Design review of the part built by this model. Coordinates are the model's own, in mm. Face numbers are marked on the shaded views. A direction names the side the tool comes from. Round coordinates to 2 decimals unless told otherwise and drop trailing zeros. Loops run counter-clockwise (first coordinate to the right, second up) from the corner with the lowest first, then second, coordinate; pieces in that order, holes last. Notation, with made-up numbers: (81.5, 60.25) - (96.5, 60.25) arc R23 cw to (96.5, 97.25) - close; hole circle Ø8 at (-38, 45). An arc over 180 degrees is marked (long way). Answer as CSV lines item,"result". Start each with the question number.
(1) For the marked faces 4 and 5, list the 3-axis set-ups (+Z, -Z, +X, -X, +Y, -Y) from which the entire face can be reached by the end or side of a thin tool; tool diameter is ignored.
(2) Consider section C-C (y = 1). Give the boundary of the cut face in (x, z) (3 decimals).
(3) Consider section D-D (x = 3.25). Give the boundary of the cut face in (y, z).
(4) For P1, Ø4, axis at x = 0, z = 0, coming from the +Y side (1 decimal); P2, Ø3, axis at x = -2, y = 5, coming from the -Z side; P3, Ø8, axis at x = 6, y = 6, coming from the +Z side; P4, Ø2, axis at x = 5, y = 12, coming from the +Z side, all flat-tipped, find the tip position at first contact; note any pin that passes through.
(5) Consider section B-B (z = 0). Give the boundary of the cut face in (x, y) (3 decimals).
(6) Mouldability with a two-part tool opening along Z and no side actions: class the marked faces 1, 2 and 3 as released by +Z, released by -Z, zero draft, split by the parting line, or undercut.
(7) Wall thickness on L1, parallel to Z at x = 0, y = 7 (3 decimals); L2, parallel to Y at x = -6.5, z = -4: over which ranges is each line inside the solid? List them lowest first.
(8) Consider section A-A (x = 0). Give the boundary of the cut face in (y, z) (3 decimals), and give its area (3 significant figures).
Autodesk Inventor part; units mm, degrees
ref_plane "YZ Plane" through (0, 0, 0) normal (1, 0, 0) x (0, 1, 0)
ref_plane "XZ Plane" through (0, 0, 0) normal (0, 1, 0) x (-1, 0, 0)
ref_plane "XY Plane" through (0, 0, 0) normal (0, 0, 1) x (1, 0, 0)
sketch "Sketch1" plane through (0, 0, 0) normal (0, 1, 0) x (-1, 0, 0)
  circle A0 centre (0, 0) radius 9
  dimension "d0" = 18
extrude "Extrusion1" add sketch "Sketch1" along normal blind 1.5
sketch "Sketch2" plane through (0, 1.5, 0) normal (0, 1, 0) x (1, 0, 0)
  circle A0 centre (0, 0) radius 6.05
  dimension "d3" = 12.1
extrude "Extrusion2" add sketch "Sketch2" along normal blind 11.2
sketch "Sketch3" plane through (0, 12.7, 0) normal (0, 1, 0) x (1, 0, 0)
  circle A0 centre (0, 0) radius 9
  dimension "d6" = 18
extrude "Extrusion3" add sketch "Sketch3" along normal blind 1.5
sketch "Sketch4" plane through (0, 14.2, 0) normal (0, 1, 0) x (1, 0, 0)
  circle A0 centre (0, 0) radius 6.05
  circle A1 centre (0, 0) radius 2.625
  dimension "d9" = 5.25
extrude "Extrusion4" cut sketch "Sketch4" against normal through all contours A1
properties part number "10mm_Idle_Pulley"
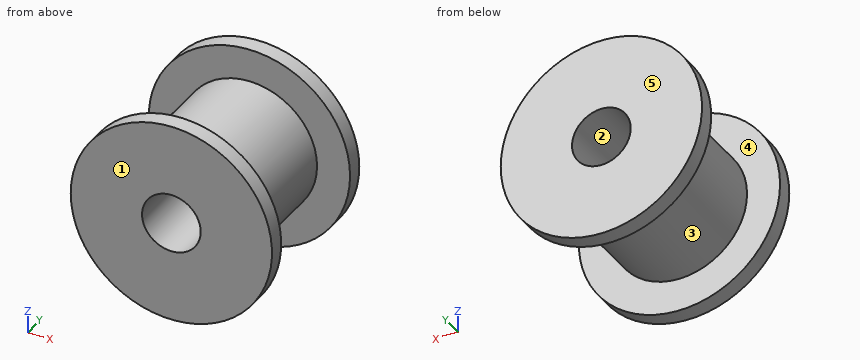
Determined:
1,face 4,"none"
1,face 5,"+Z, -Z, +X, -X, +Y"
2,outline,"circle Ø18 at (0, 0); hole circle Ø5.25 at (0, 0)"
3,outline,"(0, -8.39) - (1.5, -8.39) - (1.5, -5.1) - (12.7, -5.1) - (12.7, -8.39) - (14.2, -8.39) - (14.2, 8.39) - (12.7, 8.39) - (12.7, 5.1) - (1.5, 5.1) - (1.5, 8.39) - (0, 8.39) - close"
4,P1,"passes through"
4,P2,"stops at z = -6.03"
4,P3,"stops at z = 5.71"
4,P4,"stops at z = 7.91"
5,outline,"(-9, 0) - (-2.625, 0) - (-2.625, 14.2) - (-9, 14.2) - (-9, 12.7) - (-6.05, 12.7) - (-6.05, 1.5) - (-9, 1.5) - close; (2.625, 0) - (9, 0) - (9, 1.5) - (6.05, 1.5) - (6.05, 12.7) - (9, 12.7) - (9, 14.2) - (2.625, 14.2) - close"
6,face 1,"zero draft"
6,face 2,"undercut"
6,face 3,"split by the parting line"
7,L1,"z = -6.05 to -2.625, 2.625 to 6.05"
7,L2,"y = 0 to 1.5, 12.7 to 14.2"
8,outline,"(0, -9) - (1.5, -9) - (1.5, -6.05) - (12.7, -6.05) - (12.7, -9) - (14.2, -9) - (14.2, -2.625) - (0, -2.625) - close; (0, 2.625) - (14.2, 2.625) - (14.2, 9) - (12.7, 9) - (12.7, 6.05) - (1.5, 6.05) - (1.5, 9) - (0, 9) - close"
8,area,"115 mm^2"
